from build123d import *

# Parameters (mm, degrees)
SKETCH_W             = 132.4
SKETCH_H             = 118.2
PAD_DEPTH            = 4
PAD_DEPTH_BACK       = 10
SKETCH001_W          = 124.4
SKETCH001_H          = 114.2
POCKET_DEPTH         = 10.001
SKETCH002_W          = 116.4
SKETCH002_H          = 110.2
POCKET001_DEPTH      = 5
FILLET_R             = 6
FILLET001_R          = 10
FILLET002_R          = 2
POCKET002_DEPTH      = 10.001
POCKET002_DEPTH_BACK = 4.001
PAD001_DEPTH         = 10
SKETCH005_W          = 1
SKETCH005_H          = 8
POCKET003_DEPTH      = 10.001
POCKET003_DEPTH_BACK = 4.001
SKETCH006_R          = 1.65
POCKET004_DEPTH      = 66.201
POCKET004_DEPTH_BACK = 66.201
POCKET005_DEPTH      = 64.5
SKETCH008_R          = 1.65
POCKET006_DEPTH      = 59.101
POCKET006_DEPTH_BACK = 59.101
POCKET007_DEPTH      = 57.4


with BuildPart() as part:
    # Sketch → Pad (new body, two sides)
    with BuildSketch(Plane.XY) as pad_sk:
        Rectangle(SKETCH_W, SKETCH_H)
    extrude(amount=PAD_DEPTH)
    extrude(pad_sk.sketch, amount=-PAD_DEPTH_BACK)

    # Sketch001 → Pocket (cut, through all)
    with BuildSketch(Plane.XY):
        with Locations((0, -2)):
            Rectangle(SKETCH001_W, SKETCH001_H)
    extrude(amount=-POCKET_DEPTH, mode=Mode.SUBTRACT)

    # Sketch002 → Pocket001 (cut)
    with BuildSketch(Plane.XY):
        with Locations((0, -4)):
            Rectangle(SKETCH002_W, SKETCH002_H)
    extrude(amount=POCKET001_DEPTH, mode=Mode.SUBTRACT)

    # Fillet
    fillet_edges = [part.edges().sort_by_distance(p)[0] for p in [
        (-62.2, 55.1, -5),
        (62.2, 55.1, -5),
    ]]
    fillet(fillet_edges, radius=FILLET_R)

    # Fillet001
    fillet001_edges = [part.edges().sort_by_distance(p)[0] for p in [
        (-66.2, 59.1, -3),
        (66.2, 59.1, -3),
    ]]
    fillet(fillet001_edges, radius=FILLET001_R)

    # Fillet002
    fillet002_edges = [part.edges().sort_by_distance(p)[0] for p in [
        (-58.2, 51.1, 2),
        (58.2, 51.1, 2),
    ]]
    fillet(fillet002_edges, radius=FILLET002_R)

    # Sketch003 → Pocket002 (cut, two sides)
    with BuildSketch(Plane.XY) as pocket002_sk:
        with BuildLine():
            Line((-65.2, 39.1), (-65.2, 49.1))
            ThreePointArc((-56.2, 58.1), (-62.563961, 55.463961), (-65.2, 49.1))
            Line((-46.2, 58.1), (-56.2, 58.1))
            Line((-46.2, 58.1), (-46.2, 59.1))
            Line((-46.2, 59.1), (-56.2, 59.1))
            ThreePointArc((-56.2, 59.1), (-63.271068, 56.171068), (-66.2, 49.1))
            Line((-66.2, 39.1), (-66.2, 49.1))
            Line((-65.2, 39.1), (-66.2, 39.1))
        make_face()
        with BuildLine():
            Line((65.2, 39.1), (65.2, 49.1))
            ThreePointArc((65.2, 49.1), (62.563961, 55.463961), (56.2, 58.1))
            Line((46.2, 58.1), (56.2, 58.1))
            Line((46.2, 58.1), (46.2, 59.1))
            Line((46.2, 59.1), (56.2, 59.1))
            ThreePointArc((66.2, 49.1), (63.271068, 56.171068), (56.2, 59.1))
            Line((66.2, 39.1), (66.2, 49.1))
            Line((65.2, 39.1), (66.2, 39.1))
        make_face()
    extrude(amount=-POCKET002_DEPTH, mode=Mode.SUBTRACT)
    extrude(pocket002_sk.sketch, amount=POCKET002_DEPTH_BACK, mode=Mode.SUBTRACT)

    # Sketch004 → Pad001 (join)
    with BuildSketch(Plane.XY):
        Polygon((-62.2, 24.7), (-62.2, 26.1), (-60.55, 27), (-60.55, 23.8), align=None)
        Polygon((-62.2, 5.7), (-60.55, 4.8), (-60.55, 8), (-62.2, 7.1), align=None)
        Polygon((-62.2, -50.3), (-60.55, -51.2), (-60.55, -48), (-62.2, -48.9), align=None)
        Polygon((62.2, 24.7), (62.2, 26.1), (60.55, 27), (60.55, 23.8), align=None)
        Polygon((62.2, 5.7), (60.55, 4.8), (60.55, 8), (62.2, 7.1), align=None)
        Polygon((62.2, -50.3), (60.55, -51.2), (60.55, -48), (62.2, -48.9), align=None)
    extrude(amount=-PAD001_DEPTH)

    # Sketch005 → Pocket003 (cut, two sides)
    with BuildSketch(Plane.XY) as pocket003_sk:
        with Locations((-65.7, -55.1)):
            Rectangle(SKETCH005_W, SKETCH005_H)
        with Locations((65.7, -55.1)):
            Rectangle(SKETCH005_W, SKETCH005_H)
    extrude(amount=-POCKET003_DEPTH, mode=Mode.SUBTRACT)
    extrude(pocket003_sk.sketch, amount=POCKET003_DEPTH_BACK, mode=Mode.SUBTRACT)

    # Sketch006 → Pocket004 (cut, two sides)
    with BuildSketch(Plane.YZ) as pocket004_sk:
        with Locations((-55.1, -4)):
            Circle(SKETCH006_R)
        with Locations((44.1, -4)):
            Circle(SKETCH006_R)
    extrude(amount=-POCKET004_DEPTH, mode=Mode.SUBTRACT)
    extrude(pocket004_sk.sketch, amount=POCKET004_DEPTH_BACK, mode=Mode.SUBTRACT)

    # Sketch007 → Pocket005 (cut, symmetric)
    with BuildSketch(Plane.YZ):
        Polygon((-57.975, -5.659882), (-55.1, -7.319764), (-52.225, -5.659882), (-52.225, -2.340118), (-55.1, -0.680236), (-57.975, -2.340118), align=None)
        Polygon((44.1, -7.319764), (46.975, -5.659882), (46.975, -2.340118), (44.1, -0.680236), (41.225, -2.340118), (41.225, -5.659882), align=None)
    extrude(amount=POCKET005_DEPTH, both=True, mode=Mode.SUBTRACT)

    # Sketch008 → Pocket006 (cut, two sides)
    with BuildSketch(Plane.XZ) as pocket006_sk:
        with Locations((-51.2, -4)):
            Circle(SKETCH008_R)
        with Locations((51.2, -4)):
            Circle(SKETCH008_R)
    extrude(amount=-POCKET006_DEPTH, mode=Mode.SUBTRACT)
    extrude(pocket006_sk.sketch, amount=POCKET006_DEPTH_BACK, mode=Mode.SUBTRACT)

    # Sketch009 → Pocket007 (cut)
    with BuildSketch(Plane.XZ):
        Polygon((-51.2, -7.319764), (-48.325, -5.659882), (-48.325, -2.340118), (-51.2, -0.680236), (-54.075, -2.340118), (-54.075, -5.659882), align=None)
        Polygon((51.2, -7.319764), (54.075, -5.659882), (54.075, -2.340118), (51.2, -0.680236), (48.325, -2.340118), (48.325, -5.659882), align=None)
    extrude(amount=-POCKET007_DEPTH, mode=Mode.SUBTRACT)


solid = part.part
CAD build for the part. Positions are in the model's coordinates, mm. A direction names the side the tool comes from. Coordinates: 2 decimals unless noted, no trailing zeros. Write each loop counter-clockwise with the first axis right and the second up, starting at its lowest first coordinate (ties: lowest second). Pieces come first, ordered by that corner, then holes. Notation, with made-up numbers: (29.5, 38.5) - (37.5, 38.5) arc R20 cw to (37.5, 60.5) - close; hole circle Ø7 at (-8, -18.75). An arc over 180 degrees is marked (long way). Use a Markdown table: item, result. Add a question column.
Item 1: Mould opens along Z. For faces 1 (the face through (58.2, -6, 2)), 2 (the face through (-64.5, -56.4, -5.4)) say: pulls with the +Z half, pulls with the -Z half, needs draft (parallel to the pull), parting line crosses it, or undercut.
Item 2: Drill centre lines: L1, parallel to Z at x = -51.2, y = 57.8; L2, parallel to X at y = -23, z = -7; L3, parallel to X at y = -48.5, z = -0.5. Where is each one in solid material? Low to high. Write a range as from..to.
Item 3: 3-axis set-ups, long thin cutter, end or side, ignore diameter. For faces 3 (the face through (65.2, 44, -2)), 4 (the face through (62.2, -22, -5)), 5 (the face through (-65.2, -55, -2)): which of +Z, -Z, +X, -X, +Y, -Y reach the whole face in a straight line?
Item 4: Flat gauge pins, fed straight in: pin 1 (3 mm diameter, centred on x = 9, z = -7, fed in from -Y); pin 2 (5.5 mm diameter, centred on y = 44.1, z = -4, fed in from +X); pin 3 (5 mm diameter, centred on y = 43.5, z = -2.5, fed in from -X). Where does each tip first touch, or does it go through?
Item 5: Band-saw the part on A-A, the plane y = 30. Give the cut face in (x, z), and give its area (3 significant figures).
Item 6: Band-saw the part on C-C, the plane z = -4. Give the number of separate pieces and of enclosed holes in the cut face, and give its area (3 significant figures).
Item 7: Band-saw the part on B-B, the plane x = 16.5. Give the cut face in (y, z), and give its area (3 significant figures).
Numbers:
| question | item | result |
|---|---|---|
| 1 | face 1 | needs draft |
| 1 | face 2 | undercut |
| 2 | L1 | -10..-5.65, -2.35..4 |
| 2 | L2 | -66.2..-62.2, 62.2..66.2 |
| 2 | L3 | -66.2..-62.2, -61.47..-60.55, 60.55..61.47, 62.2..66.2 |
| 3 | face 3 | +Z, -Z, +X, +Y |
| 3 | face 4 | -Z |
| 3 | face 5 | +Z, -Z, -X, -Y |
| 4 | pin 1 | y = 55.1 |
| 4 | pin 2 | x = 65.2 |
| 4 | pin 3 | x = -65.2 |
| 5 | outline | (-66.2, -10) - (-62.2, -10) - (-62.2, 0) - (-58.2, 0) - (-58.2, 4) - (-66.2, 4) - close; (58.2, 0) - (62.2, 0) - (62.2, -10) - (66.2, -10) - (66.2, 4) - (58.2, 4) - close |
| 5 | area | 144 mm2 |
| 6 | separate pieces | 7 |
| 6 | enclosed holes | 0 |
| 6 | area | 1,260 mm2 |
| 7 | outline | (51.1, 0) - (55.1, 0) - (55.1, -10) - (59.1, -10) - (59.1, 4) - (51.1, 4) - close |
| 7 | area | 72.0 mm2 |
